Check sheet for the modelled part. Datum: model origin and axes. Units: mm. Face numbers are marked on the shaded views. Coordinates: 2 decimals unless noted, no trailing zeros. Loops run counter-clockwise (first coordinate to the right, second up) from the corner with the lowest first, then second, coordinate; pieces in that order, holes last. Notation, with made-up numbers: (-14.75, 0) -> (-2.75, 0) arc R19 cw to (-2.75, 13) -> close; hole circle Ø11 at (-16, -4). An arc over 180 degrees is marked (long way). Use CSV: the item, a comma, the result in double quotes.
```python
from build123d import *

# Parameters (mm, degrees)
SKETCH1_R           = 16.75
BOSS_EXTRUDE1_DEPTH = 3.5
SKETCH2_OUTSIDE_W   = 45.002
SKETCH2_OUTSIDE_H   = 45.002
SKETCH2_OUTSIDE_R   = 15.8
CUT_EXTRUDE1_DEPTH  = 1.5
SKETCH3_R           = 3.3
SKETCH3_R_2         = 2.2
CUT_EXTRUDE2_DEPTH  = 24.945250051


with BuildPart() as part:
    # Sketch1 → Boss-Extrude1 (new body)
    with BuildSketch(Plane(origin=(0, 0, 0), x_dir=(1, 0, 0), z_dir=(0, 1, 0))):
        with Locations(Location((0, 0, 0), (0, 0, 270))):
            Circle(SKETCH1_R)
    extrude(amount=BOSS_EXTRUDE1_DEPTH)

    # Sketch2 outside → Cut-Extrude1 (cut)
    with BuildSketch(Plane(origin=(0, 3.5, 0), x_dir=(1, 0, 0), z_dir=(0, 1, 0))):
        Rectangle(SKETCH2_OUTSIDE_W, SKETCH2_OUTSIDE_H)
        with Locations(Location((0, 0, 0), (0, 0, 270))):
            Circle(SKETCH2_OUTSIDE_R, mode=Mode.SUBTRACT)
    extrude(amount=-CUT_EXTRUDE1_DEPTH, mode=Mode.SUBTRACT)

    # Sketch3 → Cut-Extrude2 (cut, through all)
    with BuildSketch(Plane(origin=(0, 3.5, 0), x_dir=(1, 0, 0), z_dir=(0, 1, 0))):
        with Locations(Location((0, 0, 0), (0, 0, 270))):
            Circle(SKETCH3_R)
        with Locations(Location((-8.3, 0, 0), (0, 0, 270))):
            Circle(SKETCH3_R_2)
        with Locations(Location((8.3, 0, 0), (0, 0, 270))):
            Circle(SKETCH3_R_2)
    extrude(amount=-CUT_EXTRUDE2_DEPTH, mode=Mode.SUBTRACT)


solid = part.part
```
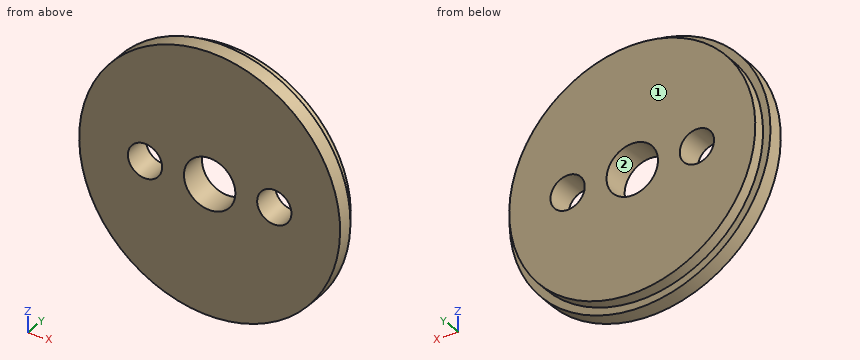
1) Cross-section at C-C on y = 2.7. Record the boundary of the cut face in (x, z).
Answer below:
outline,"circle Ø31.6 at (0, 0); hole circle Ø4.4 at (-8.3, 0); hole circle Ø6.6 at (0, 0); hole circle Ø4.4 at (8.3, 0)"
2) Thickness scan on line 1 along X through (y, z) = (0.7, 0); line 2 along X through (y, z) = (2.2, 0); line 3 along Y through (x, z) = (-11.5, 12). Record the ranges inside material, lowest first. Write a range as from..to.
Answer below:
line 1,"x = -16.75..-10.5, -6.1..-3.3, 3.3..6.1, 10.5..16.75"
line 2,"x = -15.8..-10.5, -6.1..-3.3, 3.3..6.1, 10.5..15.8"
line 3,"y = 0..2"
3) Draft check along Z on the marked faces 1 and 2. Enter one of: released by +Z, released by -Z, zero draft, split by the parting line, or undercut.
Answer below:
face 1,"zero draft"
face 2,"undercut"
4) Go/stop test with a flat-tipped pin: pin 1 Ø1.5 at (y, z) = (3, -2) entering from +X. Record where the tip stops, or that it passes through.
Answer below:
pin 1,"stops at x = 15.75"
5) Cross-section at A-A on x = 0. Record the boundary of the cut face in (y, z).
Answer below:
outline,"(0, -16.75) -> (2, -16.75) -> (2, -15.8) -> (3.5, -15.8) -> (3.5, -3.3) -> (0, -3.3) -> close; (0, 3.3) -> (3.5, 3.3) -> (3.5, 15.8) -> (2, 15.8) -> (2, 16.75) -> (0, 16.75) -> close"
6) Cross-section at D-D on z = -4. Record the boundary of the cut face in (x, y), and give its area (3 significant figures).
Answer below:
outline,"(-16.27, 0) -> (16.27, 0) -> (16.27, 2) -> (15.29, 2) -> (15.29, 3.5) -> (-15.29, 3.5) -> (-15.29, 2) -> (-16.27, 2) -> close"
area,"111 mm²"
7) Cross-section at B-B on z = 0. Record the boundary of the cut face in (x, y), and give its area (3 significant figures).
Answer below:
outline,"(-16.75, 0) -> (-10.5, 0) -> (-10.5, 3.5) -> (-15.8, 3.5) -> (-15.8, 2) -> (-16.75, 2) -> close; (-6.1, 0) -> (-3.3, 0) -> (-3.3, 3.5) -> (-6.1, 3.5) -> close; (3.3, 0) -> (6.1, 0) -> (6.1, 3.5) -> (3.3, 3.5) -> close; (10.5, 0) -> (16.75, 0) -> (16.75, 2) -> (15.8, 2) -> (15.8, 3.5) -> (10.5, 3.5) -> close"
area,"60.5 mm²"
